Geometry check sheet. Reference: the model listing, model coordinates, mm. A direction names the side the tool comes from. Round coordinates to 2 decimals unless told otherwise and drop trailing zeros. Write each loop counter-clockwise with the first axis right and the second up, starting at its lowest first coordinate (ties: lowest second). Pieces come first, ordered by that corner, then holes. Notation, with made-up numbers: (-37, 10) -> (-28, 10) arc R15 cw to (-28, 21) -> close; hole circle Ø10 at (60.25, 85). An arc over 180 degrees is marked (long way). One line per question, with ' | ' between items.
```python
from build123d import *

# Parameters (mm, degrees)
SKETCH_W        = 82.95665
SKETCH_H        = 67.908462
SKETCH_R        = 1.357232
PAD_DEPTH       = 2
SKETCH001_R     = 3.013294
SKETCH001_R_2   = 1.357232
PAD001_DEPTH    = 2
SKETCH002_W     = 86.95665
SKETCH002_H     = 71.908462
SKETCH002_W_2   = 82.95665
SKETCH002_H_2   = 67.908462
PAD002_DEPTH    = 15
SKETCH003_W     = 23.303855
SKETCH003_H     = 2
POCKET_DEPTH    = 15
SKETCH004_W     = 9.816747
SKETCH004_H     = 53.650996
SKETCH004_W_2   = 9.816748
SKETCH004_W_3   = 15.848155
POCKET001_DEPTH = 6
SKETCH006_R     = 2.929585
POCKET002_DEPTH = 43.398659
SKETCH007_W     = 66.912369
SKETCH007_H     = 53.325719
POCKET003_DEPTH = 5


with BuildPart() as part:
    # Sketch → Pad (new body)
    with BuildSketch(Plane.XY):
        with Locations((-0.079666, 0.057701)):
            Rectangle(SKETCH_W, SKETCH_H)
        with Locations((-37.482224, -29.963587)):
            Circle(SKETCH_R, mode=Mode.SUBTRACT)
        with Locations((37.52877, -29.963587)):
            Circle(SKETCH_R, mode=Mode.SUBTRACT)
        with Locations((-37.754868, 30.081388)):
            Circle(SKETCH_R, mode=Mode.SUBTRACT)
        with Locations((37.458336, 30.081388)):
            Circle(SKETCH_R, mode=Mode.SUBTRACT)
    extrude(amount=PAD_DEPTH)

    # Sketch001 (on DatumPlane) → Pad001 (join)
    with BuildSketch(Plane.XY.offset(2)):
        with Locations((-37.754868, 30.081388)):
            Circle(SKETCH001_R)
        with Locations((-37.754868, 30.081388)):
            Circle(SKETCH001_R_2, mode=Mode.SUBTRACT)
        with Locations((37.458336, 30.081388)):
            Circle(SKETCH001_R)
        with Locations((37.458336, 30.081388)):
            Circle(SKETCH001_R_2, mode=Mode.SUBTRACT)
        with Locations((37.52877, -29.963587)):
            Circle(SKETCH001_R)
        with Locations((37.52877, -29.963587)):
            Circle(SKETCH001_R_2, mode=Mode.SUBTRACT)
        with Locations((-37.482224, -29.963587)):
            Circle(SKETCH001_R)
        with Locations((-37.482224, -29.963587)):
            Circle(SKETCH001_R_2, mode=Mode.SUBTRACT)
    extrude(amount=PAD001_DEPTH)

    # Sketch002 → Pad002 (join)
    with BuildSketch(Plane.XY):
        with Locations((-0.079666, 0.057701)):
            Rectangle(SKETCH002_W, SKETCH002_H)
        with Locations((-0.079666, 0.057701)):
            Rectangle(SKETCH002_W_2, SKETCH002_H_2, mode=Mode.SUBTRACT)
    extrude(amount=PAD002_DEPTH)

    # Sketch003 (on DatumPlane) → Pocket (cut)
    with BuildSketch(Plane.XY.offset(2)):
        with Locations((-1.558922, 35.011932)):
            Rectangle(SKETCH003_W, SKETCH003_H)
    extrude(amount=POCKET_DEPTH, mode=Mode.SUBTRACT)

    # Sketch004 (on DatumPlane) → Pocket001 (cut)
    with BuildSketch(Plane(origin=(37.458336, 30.081388, 6), x_dir=(0, 1, 0), z_dir=(0, 0, 1))):
        with Locations((-41.548102, 54.190829)):
            Rectangle(SKETCH004_W, SKETCH004_H)
        with Locations((-27.168644, 54.190829)):
            Rectangle(SKETCH004_W_2, SKETCH004_H)
        with Locations((-12.643048, 54.190829)):
            Rectangle(SKETCH004_W_3, SKETCH004_H)
    extrude(amount=POCKET001_DEPTH, mode=Mode.SUBTRACT)

    # Sketch006 → Pocket002 (cut)
    with BuildSketch(Plane.YZ):
        with Locations((10.200474, 8.212474)):
            Circle(SKETCH006_R)
        with Locations((20.473468, 8.212474)):
            Circle(SKETCH006_R)
    extrude(amount=POCKET002_DEPTH, mode=Mode.SUBTRACT)

    # Sketch007 → Pocket003 (cut)
    with BuildSketch(Plane.XY):
        with Locations((0.089973, -0.812508)):
            Rectangle(SKETCH007_W, SKETCH007_H)
    extrude(amount=POCKET003_DEPTH, mode=Mode.SUBTRACT)


solid = part.part
```
(1) Sectioned sample at A-A on x = 19. Record the cut outline in (y, z), then the cut area to 3 significant figures.
Resolved:
outline: (-35.9, 0) -> (-27.48, 0) -> (-27.48, 2) -> (-33.9, 2) -> (-33.9, 15) -> (-35.9, 15) -> close; (25.85, 0) -> (36.01, 0) -> (36.01, 15) -> (34.01, 15) -> (34.01, 2) -> (25.85, 2) -> close | area: 89.2 mm2
(2) Sectioned sample at B-B on y = 0. Record the cut outline in (x, z).
Resolved:
outline: (-43.56, 0) -> (-33.37, 0) -> (-33.37, 2) -> (-41.56, 2) -> (-41.56, 6) -> (-43.56, 6) -> close; (-43.56, 12) -> (-41.56, 12) -> (-41.56, 15) -> (-43.56, 15) -> close; (33.55, 0) -> (43.4, 0) -> (43.4, 15) -> (41.4, 15) -> (41.4, 2) -> (33.55, 2) -> close
(3) Go/stop test with flat-tipped pins: pin 1 (3 mm diameter, centred on x = -38.5, y = 29.5, fed in from +Z); pin 2 (1 mm diameter, centred on x = -43, y = 4.5, fed in from -Z); pin 3 (6.5 mm diameter, centred on x = -6, z = 6, fed in from +Y). Record where each tip stops, or that it passes through.
Resolved:
pin 1: stops at z = 4 | pin 2: stops at z = 0 | pin 3: stops at y = -33.9
(4) Sectioned sample at C-C on z = 7. Count the separate pieces of the cut face and the enclosed holes in it, then the cut area to 3 significant figures.
Resolved:
separate pieces: 6 | enclosed holes: 0 | area: 481 mm2
(5) Material ranges on line 1 (X direction, y = -17, z = 10.75); line 2 (Y direction, x = 33, z = 14); line 3 (X direction, y = -6.5, z = 1.75), recorded low to high.
Resolved:
line 1: x = -43.56 to -41.56, 41.4 to 43.4 | line 2: y = -35.9 to -33.9, 34.01 to 36.01 | line 3: x = -43.56 to -33.37, 33.55 to 43.4
(6) Access from +Z, -Z, +X, -X, +Y, -Y to the whole of each face (thin tool, end or side, straight path). Record for faces 4 (the cylindrical face through (-34.97, 28.93, 2.99)), 5 (the flat face through (0, 25.85, 1)), 6 (the flat face through (-43, -1.996, 9)), 7 (the cylindrical face through (42.385, 12.995, 9.092)).
Resolved:
face 4: +Z | face 5: +Z, -Z | face 6: -X | face 7: +X
(7) Sectioned sample at D-D on x = 9. Record the cut outline in (y, z).
Resolved:
outline: (-35.9, 0) -> (-27.48, 0) -> (-27.48, 2) -> (-33.9, 2) -> (-33.9, 15) -> (-35.9, 15) -> close; (25.85, 0) -> (36.01, 0) -> (36.01, 2) -> (25.85, 2) -> close
(8) Draft check along X on faces 1 (the cylindrical face through (42.385, 17.547, 8.341)), 2 (the flat face through (41.399, 0, 8)), 3 (the flat face through (43.399, 0, 7)). Enter one of: +X half, -X half, draft (parallel to the pull), parting line (faces both ways), or undercut.
Resolved:
face 1: draft | face 2: undercut | face 3: +X half
